from build123d import *

# Parameters (mm, degrees)
F1_DEPTH      = 15
F2_T1_DEPTH   = 25
F2_T3_DEPTH   = 24.6824583655
F3_R          = 0.25
F6_DEPTH      = 5
F7_R          = 3.5
F8_DEPTH      = 7.501
F8_DEPTH_BACK = 7.501


# Not quite as in the source:
# - a fillet or chamfer that OpenCascade refuses, or shapes differently, is made with other operations: its cross-section is extruded or revolved along the edge and cut away or added
# - a feature names something its author has since deleted; it is built from what else it names


with BuildPart() as f1:
    # F0 (on Top) → F1 (new body)
    with BuildSketch(Plane.XY):
        with BuildLine():
            Line((3, 11.8), (0, 11.8))
            Line((0, 11.8), (0, 0))
            Line((0, 0), (11.8, 0))
            Line((11.8, 0), (11.8, 3))
            Line((11.8, 3), (11.8, 6))
            Line((11.8, 6), (10.3, 6))
            Line((10.3, 6), (8.8, 4.5))
            Line((8.8, 4.5), (10.3, 4.5))
            Line((10.3, 4.5), (10.3, 3))
            Line((10.3, 3), (3.5, 3))
            ThreePointArc((3.5, 3), (2.6464466094, 2.6464466094), (3, 3.5))
            Line((3, 3.5), (3, 10.3))
            Line((3, 10.3), (4.5, 10.3))
            Line((4.5, 10.3), (4.5, 8.8))
            Line((4.5, 8.8), (6, 10.3))
            Line((6, 10.3), (6, 11.8))
            Line((6, 11.8), (3, 11.8))
        make_face()
    extrude(amount=F1_DEPTH)

    # F2: fillet of radius 2 on 4 edges, made by hand

    # F2_s2 → F2_t1 (cut)
    with BuildSketch(Plane.XY.offset(-5)):
        with BuildLine():
            ThreePointArc((2, 11.8), (0.5857864376, 11.2142135624), (0, 9.8))
            Line((0, 9.8), (0, 11.8))
            Line((0, 11.8), (2, 11.8))
        make_face()
        with BuildLine():
            ThreePointArc((11.8, 2), (11.2142135624, 0.5857864376), (9.8, 0))
            Line((9.8, 0), (11.8, 0))
            Line((11.8, 0), (11.8, 2))
        make_face()
    extrude(amount=F2_T1_DEPTH, mode=Mode.SUBTRACT)

    # F2_s4 → F2_t3 (cut)
    with BuildSketch(Plane.XY.offset(-4.8412291828)):
        with BuildLine():
            ThreePointArc((4.0635083269, 11.8), (5.2882531983, 11.3811388301), (6, 10.3))
            Line((6, 10.3), (6, 11.8))
            Line((6, 11.8), (4.0635083269, 11.8))
        make_face()
        with BuildLine():
            ThreePointArc((10.3, 6), (11.3811388301, 5.2882531983), (11.8, 4.0635083269))
            Line((11.8, 4.0635083269), (11.8, 6))
            Line((11.8, 6), (10.3, 6))
        make_face()
    extrude(amount=F2_T3_DEPTH, mode=Mode.SUBTRACT)

    # F3
    f3_edges = [f1.edges().sort_by_distance(p)[0] for p in [
        (3, 10.3, 7.5),
        (4.5, 10.3, 7.5),
        (4.5, 8.8, 7.5),
        (3, 3.5, 7.5),
        (3.5, 3, 7.5),
        (10.3, 4.5, 7.5),
        (8.8, 4.5, 7.5),
        (10.3, 3, 7.5),
    ]]
    fillet(f3_edges, radius=F3_R)

    # F5 (on mid) → F6 (join, symmetric)
    with BuildSketch(Plane.XY.offset(7.5)):
        with BuildLine():
            ThreePointArc((-0.9090909212, 2.1252021099), (-0.2326870569, 3.4924432671), (0, 5))
            ThreePointArc((0, 5), (-0.2326870569, 6.5075567329), (-0.9090909212, 7.8747978901))
            ThreePointArc((-0.9090909212, 7.8747978901), (-10, 5), (-0.9090909212, 2.1252021099))
        make_face()
        with BuildLine():
            Line((0, 1.8377223398), (0, 5))
            ThreePointArc((0, 5), (-0.2326870569, 3.4924432671), (-0.9090909212, 2.1252021099))
            ThreePointArc((-0.9090909212, 2.1252021099), (-0.3492443377, 2.3144536376), (0, 1.8377223398))
        make_face()
        with BuildLine():
            ThreePointArc((-0.9090909212, 7.8747978901), (-0.2326870569, 6.5075567329), (0, 5))
            Line((0, 5), (0, 8.1622776602))
            ThreePointArc((0, 8.1622776602), (-0.3492443377, 7.6855463624), (-0.9090909212, 7.8747978901))
        make_face()
    extrude(amount=F6_DEPTH, both=True)

    # F7 (on mid) → F8 (cut, two sides)
    with BuildSketch(Plane.XY.offset(7.5)) as f8_sk:
        with Locations((-5, 5)):
            Circle(F7_R)
    extrude(amount=-F8_DEPTH, mode=Mode.SUBTRACT)
    extrude(f8_sk.sketch, amount=F8_DEPTH_BACK, mode=Mode.SUBTRACT)


solid = f1.part
Verification items for the finished model (mm, model axes). A direction names the side the tool comes from. Give positions to 0.01 mm unless a question says otherwise; leave off trailing zeros. Loops run counter-clockwise (first coordinate to the right, second up) from the corner with the lowest first, then second, coordinate; pieces in that order, holes last.
1. Material ranges on probe 1 along Y at (x, z) = (-5, 11); probe 2 along X at (y, z) = (5, 11.3); probe 3 along Z at (x, y) = (-8.25, 2), recorded low to high.
Derived:
probe 1: y = 0 to 1.5, 8.5 to 10
probe 2: x = -10 to -8.5, -1.5 to 3, 9.3 to 11.57
probe 3: z = 2.5 to 12.5
2. Cross-section at B-B on z = 1.5. Record the cut outline in (x, y), and give its area (3 significant figures).
Derived:
outline: (0, 0) - (9.8, 0) arc R2 ccw to (11.8, 2) - (11.8, 4.06) arc R2 ccw to (10.3, 6) - (9.23, 4.93) arc R0.25 ccw to (9.4, 4.5) - (10.05, 4.5) arc R0.25 cw to (10.3, 4.25) - (10.3, 3.25) arc R0.25 cw to (10.05, 3) - (3.71, 3) arc R0.25 ccw to (3.47, 2.83) arc R0.5 cw (long way) to (2.83, 3.47) arc R0.25 ccw to (3, 3.71) - (3, 10.05) arc R0.25 cw to (3.25, 10.3) - (4.25, 10.3) arc R0.25 cw to (4.5, 10.05) - (4.5, 9.4) arc R0.25 ccw to (4.93, 9.23) - (6, 10.3) arc R2 ccw to (4.06, 11.8) - (2, 11.8) arc R2 ccw to (0, 9.8) - close
area: 69.1 mm2
3. Cross-section at C-C on y = 7. Record the cut outline in (x, z), and give its area (3 significant figures).
Derived:
outline: (-9.58, 2.5) - (-7.87, 2.5) - (-7.87, 12.5) - (-9.58, 12.5) - close; (-2.13, 2.5) - (0, 2.5) - (0, 0) - (3, 0) - (3, 15) - (0, 15) - (0, 12.5) - (-2.13, 12.5) - close
area: 83.4 mm2
4. Tool access check on faces 1 (the flat face through (7, 3, 7)), 2 (the flat face through (-2.8, 1.7, 12.5)), 3 (the flat face through (5.5, 9.8, 7.4)). Record the directions out of +Z, -Z, +X, -X, +Y, -Y that give a thin tool (end or side, any length) a straight path to the whole face; none if there is none.
Derived:
face 1: +Z, -Z
face 2: +Z, -X, +Y, -Y
face 3: +Z, -Z, +X
5. Go/stop test with flat-tipped pins: P1, Ø6, axis at y = 10, z = 4.5, coming from the +X side; P2, Ø2, axis at x = -4, y = 10, coming from the -Z side; P3, Ø4, axis at x = -7.5, z = 9.5, coming from the -Y side. Record where each tip stops, or that it passes through.
Derived:
P1: stops at x = 6
P2: stops at z = 2.5
P3: stops at y = 0.03
6. Cross-section at A-A on x = -5. Record the cut outline in (y, z).
Derived:
outline: (0, 2.5) - (1.5, 2.5) - (1.5, 12.5) - (0, 12.5) - close; (8.5, 2.5) - (10, 2.5) - (10, 12.5) - (8.5, 12.5) - close
7. Release check for a two-part mould opening along Y. For faces 4 (the cylindrical face through (11.37, 5.3, 7.39)), 5 (the cylindrical face through (2.7, 2.6, 7.4)), 6 (the flat face through (5, 2, 0)) record: +Y half, -Y half, draft (parallel to the pull), parting line (faces both ways), or undercut.
Derived:
face 4: +Y half
face 5: undercut
face 6: draft
